from build123d import *

# Parameters (mm, degrees)
SKETCH1_R            = 10
BOSS_EXTRUDE1_DEPTH  = 12
SKETCH2_R            = 17.55
CUT_EXTRUDE1_DEPTH   = 3
CUT_EXTRUDE2_DEPTH   = 12
SKETCH4_R            = 4
CUT_EXTRUDE3_DEPTH   = 12
SKETCH5_R            = 16.05
CUT_EXTRUDE4_DEPTH   = 113.720894248
CUT_EXTRUDE6_DEPTH   = 8
CUT_EXTRUDE7_DEPTH   = 3
SKETCH11_R           = 4.2
BOSS_EXTRUDE2_DEPTH  = 12
CUT_EXTRUDE_1_DEPTH  = 151.685102117
SKETCH_1_R           = 4.5
CUT_EXTRUDE_4_DEPTH  = 151.894002532
SKETCH6_W            = 55
SKETCH6_H            = 45.3
CUT_EXTRUDE_6_DEPTH  = 5
SKETCH_6_R           = 1.25
CUT_EXTRUDE_9_DEPTH  = 3
SKETCH_7_R           = 1.5
CUT_EXTRUDE_10_DEPTH = 151.894002532
CUT_EXTRUDE_11_DEPTH = 2.5
FILLET_1_R           = 2
FILLET_2_R           = 2
SKETCH_8_W           = 2
SKETCH_8_H           = 7.197706212
CUT_EXTRUDE_12_DEPTH = 2.5


with BuildPart() as part:
    # Sketch1 → Boss-Extrude1 (new body)
    with BuildSketch(Plane(origin=(0, 0, 0), x_dir=(1, 0, 0), z_dir=(0, 1, 0))):
        with BuildLine():
            Line((3.862942675, 39.81303397), (105, 30))
            Line((105, 30), (105, -30))
            Line((105, -30), (3.862942675, -39.81303397))
            ThreePointArc((3.862942675, -39.81303397), (-40, 0), (3.862942675, 39.81303397))
        make_face()
        with Locations(Location((0, 0, 0), (0, 0, 270))):
            Circle(SKETCH1_R, mode=Mode.SUBTRACT)
    extrude(amount=BOSS_EXTRUDE1_DEPTH)

    # Sketch2 → Cut-Extrude1 (cut)
    with BuildSketch(Plane(origin=(0, 12, 0), x_dir=(1, 0, 0), z_dir=(0, 1, 0))):
        with Locations(Location((0, 0, 0), (0, 0, 270))):
            Circle(SKETCH2_R)
    extrude(amount=-CUT_EXTRUDE1_DEPTH, mode=Mode.SUBTRACT)

    # Sketch3 → Cut-Extrude2 (cut)
    with BuildSketch(Plane(origin=(0, 12, 0), x_dir=(1, 0, 0), z_dir=(0, 1, 0))):
        with BuildLine():
            Line((71.3, 9.5), (83.3, 9.5))
            ThreePointArc((83.3, 9.5), (92.8, 0), (83.3, -9.5))
            Line((83.3, -9.5), (71.3, -9.5))
            ThreePointArc((71.3, -9.5), (61.8, 0), (71.3, 9.5))
        make_face()
    extrude(amount=-CUT_EXTRUDE2_DEPTH, mode=Mode.SUBTRACT)

    # Sketch4 → Cut-Extrude3 (cut)
    with BuildSketch(Plane(origin=(0, 12, 0), x_dir=(1, 0, 0), z_dir=(0, 1, 0))):
        with Locations(Location((30, 0, 0), (0, 0, 270))):
            Circle(SKETCH4_R)
        with Locations(Location((0, -30, 0), (0, 0, 270))):
            Circle(SKETCH4_R)
        with Locations(Location((-30, 0, 0), (0, 0, 270))):
            Circle(SKETCH4_R)
        with Locations(Location((0, 30, 0), (0, 0, 270))):
            Circle(SKETCH4_R)
    extrude(amount=-CUT_EXTRUDE3_DEPTH, mode=Mode.SUBTRACT)

    # Sketch5 → Cut-Extrude4 (cut, through all)
    with BuildSketch(Plane.XZ.offset(-9)):
        with Locations(Location((0, 0, 0), (0, 0, 270))):
            Circle(SKETCH5_R)
    extrude(amount=CUT_EXTRUDE4_DEPTH, mode=Mode.SUBTRACT)

    # Sketch7 → Cut-Extrude6 (cut)
    with BuildSketch(Plane(origin=(0, 12, 0), x_dir=(1, 0, 0), z_dir=(0, 1, 0))):
        Polygon((-7.505553499, 30), (-3.75277675, 23.5), (3.75277675, 23.5), (7.505553499, 30), (3.75277675, 36.5), (-3.75277675, 36.5), align=None)
        Polygon((-30, -7.505553499), (-23.5, -3.75277675), (-23.5, 3.75277675), (-30, 7.505553499), (-36.5, 3.75277675), (-36.5, -3.75277675), align=None)
        Polygon((30, 7.505553499), (23.5, 3.75277675), (23.5, -3.75277675), (30, -7.505553499), (36.5, -3.75277675), (36.5, 3.75277675), align=None)
        Polygon((7.505553499, -30), (3.75277675, -23.5), (-3.75277675, -23.5), (-7.505553499, -30), (-3.75277675, -36.5), (3.75277675, -36.5), align=None)
    extrude(amount=-CUT_EXTRUDE6_DEPTH, mode=Mode.SUBTRACT)

    # Sketch9 → Cut-Extrude7 (cut)
    with BuildSketch(Plane(origin=(0, 12, 0), x_dir=(1, 0, 0), z_dir=(0, 1, 0))):
        with BuildLine():
            Line((55.8, 20.5), (63.8, 20.5))
            ThreePointArc((63.8, 20.5), (66.8, 17.5), (63.8, 14.5))
            Line((63.8, 14.5), (55.8, 14.5))
            ThreePointArc((55.8, 14.5), (52.8, 17.5), (55.8, 20.5))
        make_face()
        with BuildLine():
            Line((90.8, 20.5), (98.8, 20.5))
            ThreePointArc((98.8, 20.5), (101.8, 17.5), (98.8, 14.5))
            Line((98.8, 14.5), (90.8, 14.5))
            ThreePointArc((90.8, 14.5), (87.8, 17.5), (90.8, 20.5))
        make_face()
        with BuildLine():
            Line((55.8, -14.5), (63.8, -14.5))
            ThreePointArc((63.8, -14.5), (66.8, -17.5), (63.8, -20.5))
            Line((63.8, -20.5), (55.8, -20.5))
            ThreePointArc((55.8, -20.5), (52.8, -17.5), (55.8, -14.5))
        make_face()
        with BuildLine():
            Line((90.8, -14.5), (98.8, -14.5))
            ThreePointArc((98.8, -14.5), (101.8, -17.5), (98.8, -20.5))
            Line((98.8, -20.5), (90.8, -20.5))
            ThreePointArc((90.8, -20.5), (87.8, -17.5), (90.8, -14.5))
        make_face()
    extrude(amount=-CUT_EXTRUDE7_DEPTH, mode=Mode.SUBTRACT)

    # Sketch11 → Boss-Extrude2 (add)
    with BuildSketch(Plane(origin=(0, 12, 0), x_dir=(1, 0, 0), z_dir=(0, 1, 0))):
        with BuildLine():
            Line((105, -30), (105, 30))
            Line((105, 30), (115, 30))
            ThreePointArc((115, 30), (145, 0), (115, -30))
            Line((115, -30), (105, -30))
        make_face()
        with Locations(Location((115, 0, 0), (0, 0, 270))):
            Circle(SKETCH11_R, mode=Mode.SUBTRACT)
    extrude(amount=-BOSS_EXTRUDE2_DEPTH)

    # Sketch10 → 切除-拉伸1 (cut, through all)
    with BuildSketch(Plane(origin=(0, 9, 0), x_dir=(1, 0, 0), z_dir=(0, 1, 0))):
        with BuildLine():
            Line((55.8, 15.6), (63.8, 15.6))
            ThreePointArc((63.8, 15.6), (65.7, 17.5), (63.8, 19.4))
            Line((63.8, 19.4), (55.8, 19.4))
            ThreePointArc((55.8, 19.4), (53.9, 17.5), (55.8, 15.6))
        make_face()
        with BuildLine():
            Line((90.8, 15.6), (98.8, 15.6))
            ThreePointArc((98.8, 15.6), (100.7, 17.5), (98.8, 19.4))
            Line((98.8, 19.4), (90.8, 19.4))
            ThreePointArc((90.8, 19.4), (88.9, 17.5), (90.8, 15.6))
        make_face()
        with BuildLine():
            Line((55.8, -19.4), (63.8, -19.4))
            ThreePointArc((63.8, -19.4), (65.7, -17.5), (63.8, -15.6))
            Line((63.8, -15.6), (55.8, -15.6))
            ThreePointArc((55.8, -15.6), (53.9, -17.5), (55.8, -19.4))
        make_face()
        with BuildLine():
            Line((90.8, -19.4), (98.8, -19.4))
            ThreePointArc((98.8, -19.4), (100.7, -17.5), (98.8, -15.6))
            Line((98.8, -15.6), (90.8, -15.6))
            ThreePointArc((90.8, -15.6), (88.9, -17.5), (90.8, -19.4))
        make_face()
    extrude(amount=-CUT_EXTRUDE_1_DEPTH, mode=Mode.SUBTRACT)

    # 草图1 → 切除-拉伸4 (cut, through all)
    with BuildSketch(Plane(origin=(0, 12, 0), x_dir=(1, 0, 0), z_dir=(0, 1, 0))):
        with Locations(Location((104.8, 0, 0), (0, 0, 270))):
            Circle(SKETCH_1_R)
    extrude(amount=-CUT_EXTRUDE_4_DEPTH, mode=Mode.SUBTRACT)

    # Sketch6 → 切除-拉伸6 (cut)
    with BuildSketch(Plane.XZ):
        with Locations((77.3, 0)):
            Rectangle(SKETCH6_W, SKETCH6_H)
    extrude(amount=-CUT_EXTRUDE_6_DEPTH, mode=Mode.SUBTRACT)

    # 草图6 → 切除-拉伸9 (cut)
    with BuildSketch(Plane(origin=(0, 12, 0), x_dir=(1, 0, 0), z_dir=(0, 1, 0))):
        with Locations(Location((7.999999657, -25, 0), (0, 0, 270))):
            Circle(SKETCH_6_R)
    extrude(amount=-CUT_EXTRUDE_9_DEPTH, mode=Mode.SUBTRACT)

    # 草图7 → 切除-拉伸10 (cut, through all)
    with BuildSketch(Plane.XZ):
        with Locations(Location((75, -27.910812583, 0), (0, 0, 270))):
            Circle(SKETCH_7_R)
        with Locations(Location((75, 27.910812583, 0), (0, 0, 270))):
            Circle(SKETCH_7_R)
        with Locations(Location((52.460378125, -30.097766416, 0), (0, 0, 270))):
            Circle(SKETCH_7_R)
        with Locations(Location((52.460378125, 30.097766416, 0), (0, 0, 270))):
            Circle(SKETCH_7_R)
    extrude(amount=-CUT_EXTRUDE_10_DEPTH, mode=Mode.SUBTRACT)

    # 草图4 → 切除-拉伸11 (cut)
    with BuildSketch(Plane.XZ):
        Polygon((75, 24.735386103), (77.75, 26.323099343), (77.75, 29.498525824), (75, 31.086239064), (72.25, 29.498525824), (72.25, 26.323099343), align=None)
        Polygon((75, -31.086239064), (77.75, -29.498525824), (77.75, -26.323099343), (75, -24.735386103), (72.25, -26.323099343), (72.25, -29.498525824), align=None)
        Polygon((52.460378125, 26.922339935), (55.210378125, 28.510053176), (55.210378125, 31.685479656), (52.460378125, 33.273192896), (49.710378125, 31.685479656), (49.710378125, 28.510053176), align=None)
        Polygon((52.460378125, -33.273192896), (55.210378125, -31.685479656), (55.210378125, -28.510053176), (52.460378125, -26.922339935), (49.710378125, -28.510053176), (49.710378125, -31.685479656), align=None)
    extrude(amount=-CUT_EXTRUDE_11_DEPTH, mode=Mode.SUBTRACT)

    # 圆角1
    # the kernel refuses this fillet: 2 mm, written as the material it takes off along each edge
    with BuildSketch(Plane(origin=(3.862942675, 12, -39.81303397), x_dir=(0, -1, 0), z_dir=(0.9953258492472392, 0, 0.09657356688174112))) as fillet_1_piece_1_section:
        with BuildLine():
            CenterArc((FILLET_1_R, -FILLET_1_R), FILLET_1_R, 90, 90)
            Line((0, -FILLET_1_R), (0, 0))
            Line((0, 0), (FILLET_1_R, 0))
        make_face()
    fillet_1_piece_1 = extrude(amount=106.612007165, mode=Mode.PRIVATE)
    fillet_1_piece_1 = split(fillet_1_piece_1, bisect_by=Plane(origin=(52.168611778, 11.535533923, -30), z_dir=(0, 0, -1)), keep=Keep.TOP, mode=Mode.PRIVATE)
    add(fillet_1_piece_1, mode=Mode.SUBTRACT)
    with BuildSketch(Plane(origin=(0, 12, 0), x_dir=(0.09657356688174115, 0, 0.9953258492472392), z_dir=(0.9953258492472392, 0, -0.09657356688174115))) as fillet_1_piece_2:
        with BuildLine():
            CenterArc((40 - FILLET_1_R, FILLET_1_R), FILLET_1_R, 270, 90)
            Line((40 - FILLET_1_R, 0), (40, 0))
            Line((40, 0), (40, FILLET_1_R))
        make_face()
    revolve(axis=Axis((0, 12, 0), (0, -1, 0)), revolution_arc=191.083790079, mode=Mode.SUBTRACT)
    with BuildSketch(Plane(origin=(109.976629246, 12, 29.517132166), x_dir=(-0.09657356688174114, 0, -0.9953258492472393), z_dir=(-0.9953258492472392, 0, 0.09657356688174112))) as fillet_1_piece_3_section:
        with BuildLine():
            CenterArc((FILLET_1_R, FILLET_1_R), FILLET_1_R, 180, 90)
            Line((0, FILLET_1_R), (0, 0))
            Line((0, 0), (FILLET_1_R, 0))
        make_face()
    fillet_1_piece_3 = extrude(amount=106.612007165, mode=Mode.PRIVATE)
    fillet_1_piece_3 = split(fillet_1_piece_3, bisect_by=Plane(origin=(52.168611778, 11.535533923, 30), z_dir=(0, 0, 1)), keep=Keep.TOP, mode=Mode.PRIVATE)
    add(fillet_1_piece_3, mode=Mode.SUBTRACT)

    # 圆角2
    fillet_2_edges = [part.edges().sort_by_distance(p)[0] for p in [
        (99.645199693, 12, 30),
        (99.645199693, 12, -30),
        (145, 12, 0),
    ]]
    fillet(fillet_2_edges, radius=FILLET_2_R)

    # 草图8 → 切除-拉伸12 (cut)
    with BuildSketch(Plane.ZY.offset(40)):
        with Locations((0, 8.401146894)):
            Rectangle(SKETCH_8_W, SKETCH_8_H)
    extrude(amount=-CUT_EXTRUDE_12_DEPTH, mode=Mode.SUBTRACT)


solid = part.part
Can you work these out from the model? Positions are in its coordinate system, mm. A direction names the side the tool comes from. Coordinates: 2 decimals unless noted, no trailing zeros. Write item = value, one per line.
(1) For pin 1 Ø1.2 at (x, z) = (8.5, 25) entering from +Y; pin 2 Ø2 at (x, y) = (59, 7) entering from +Z; pin 3 Ø5 at (y, z) = (3.5, 21) entering from -X, each with a flat end and sliding along its axis, tell me the tip position at first contact or that it passes through.
Results are:
pin_1 = 9
pin_2 = 34.56
pin_3 = -35.46
(2) If we mould it in two halves opening along Z, with no side actions, what happens to faces 1 (the face through (110, 5, -30)), 2 (the face through (23.5, 8, 0))? For each: pulls with the +Z half, pulls with the -Z half, needs draft (parallel to the pull), parting line crosses it, or undercut.
Results are:
face_1 = pulls with the -Z half
face_2 = undercut
(3) I need wall thicknesses on line 1 along X through (y, z) = (4.5, 0); line 2 along X through (y, z) = (1.75, 0); line 3 along X through (y, z) = (8.25, 19). Which ranges of each line are inside material? Lowest first, please. Write a range as [from, to].
Results are:
line_1 = [-40, -36.5], [-23.5, -16.05], [16.05, 23.5], [36.5, 49.8], [109.3, 110.8], [119.2, 145]
line_2 = [-40, -34], [-26, -16.05], [16.05, 26], [34, 49.8], [109.3, 110.8], [119.2, 145]
line_3 = [-35.2, 54.63], [64.97, 89.63], [99.97, 138.22]
(4) Suppose I cut it at A-A on x = 0. State how many separate pieces and enclosed holes the cut face has, plus the area to 3 significant figures.
Results are:
separate_pieces = 4
enclosed_holes = 0
area = 292 mm2
(5) For faces 3 (the face through (51, 2.5, -31)), 4 (the face through (60, 7, 19.4)), 5 (the face through (-33.2, 8.06, -5.66)), which set-ups out of +Z, -Z, +X, -X, +Y, -Y let a thin tool reach every point of the face, with its end or its side?
Results are:
face_3 = -Y
face_4 = +Y, -Y
face_5 = +Y
